Read the model definition and answer for the solid it produces. Units are mm, in the model's axes. Face numbers are marked on the shaded views. Give positions to 0.01 mm unless a question says otherwise; leave off trailing zeros. Loops run counter-clockwise (first coordinate to the right, second up) from the corner with the lowest first, then second, coordinate; pieces in that order, holes last.
(1) Find section C-C, the plane z = 32. Write down the section's boundary in (x, y) (3 decimals), then the cut area to 3 significant figures.
(2) Determine the mould class of the marked faces 1, 2 and 3 for opening direction Y: pulls with the +Y half, pulls with the -Y half, needs draft (parallel to the pull), parting line crosses it, or undercut.
(3) Straight lines are drawn through the part: probe 1 along X at (y, z) = (0, 31) (3 decimals); probe 2 along Z at (x, y) = (5, -3); probe 3 along Y at (x, z) = (0, 5) (3 decimals). For each, find the intervals that lie inside material, in ascending order.
(4) Find section D-D, the plane x = 11.5. Write down the section's boundary in (y, z), then the cut area to 3 significant figures.
(5) Each of these flat-tipped pins is pushed along its axis until it touches: P1, Ø5, axis at x = -6, z = 23, coming from the +Y side; P2, Ø1.5, axis at y = 2.5, z = 10.5, coming from the +X side; P3, Ø5, axis at y = -8, z = 21, coming from the -X side. Where does it stop, or does it pass through?
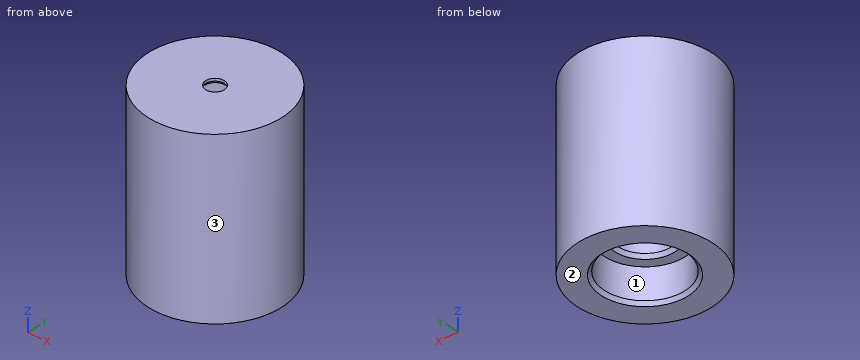
```python
from build123d import *

# Parameters (mm, degrees)
F2_SIZE2 = 0.293294
F2_SIZE  = 0.508
F3_SIZE  = 0.762


with BuildPart() as f1:
    # F0 (on Right) → F1 (revolve)
    with BuildSketch(Plane.YZ):
        Polygon((15.875, 40.64), (2.2225, 40.64), (2.2225, 39.5224), (6.35, 39.5224), (6.35, 8.0264), (9.525, 8.0264), (9.525, 0), (15.875, 0), align=None)
    revolve(axis=Axis((0, 0, 20.32), (0, 0, 1)))

    # F2
    f2_edges = [f1.edges().sort_by_distance(p)[0] for p in [
        (0, -2.2225, 39.5224),
    ]]
    chamfer(f2_edges, length=F2_SIZE, length2=F2_SIZE2)

    # F3
    f3_edges = [f1.edges().sort_by_distance(p)[0] for p in [
        (0, -6.35, 8.0264),
        (0, -9.525, 0),
    ]]
    chamfer(f3_edges, length=F3_SIZE)


solid = f1.part
```
Entries:
1. outline: circle Ø31.75 at (0, 0); hole circle Ø12.7 at (0, 0)
1. area: 665 mm2
2. face 1: undercut
2. face 2: needs draft
2. face 3: parting line crosses it
3. probe 1: x = -15.875 to -6.35, 6.35 to 15.875
3. probe 2: z = 39.52 to 40.64
3. probe 3: y = -15.875 to -9.525, 9.525 to 15.875
4. outline: (-10.94, 0) - (10.94, 0) - (10.94, 40.64) - (-10.94, 40.64) - close
4. area: 890 mm2
5. P1: stops at y = 15.48
5. P2: stops at x = 15.78
5. P3: stops at x = -14.89
